from build123d import *

# Parameters (mm, degrees)
F0_R     = 25.4
F0_R_2   = 12.7
F1_DEPTH = 3.175
F2_R     = 12.7
F3_DEPTH = 12.7
F4_R     = 7.9375
F5_DEPTH = 76.2
F7_DEPTH = 25.4
F9_DEPTH = 50.8


with BuildPart() as f1:
    # F0 (on Front) → F1 (new body)
    with BuildSketch(Plane.XZ):
        Circle(F0_R)
        Circle(F0_R_2, mode=Mode.SUBTRACT)
    extrude(amount=F1_DEPTH)

    # F2 (on Front) → F3 (join)
    with BuildSketch(Plane.XZ):
        Circle(F2_R)
    extrude(amount=F3_DEPTH)

    # F4 (on Front) → F5 (cut)
    with BuildSketch(Plane.XZ):
        Circle(F4_R)
    extrude(amount=F5_DEPTH, mode=Mode.SUBTRACT)

    # F6 (on Front) → F7 (cut)
    with BuildSketch(Plane.XZ):
        with BuildLine():
            Line((-0.1134674759, 18.3305198635), (1.9560859375, 17.1526827645))
            ThreePointArc((1.9560859375, 17.1526827645), (2.1885398686, 17.7213288028), (2.2677825241, 18.3305198635))
            ThreePointArc((2.2677825241, 18.3305198635), (-0.7368962138, 20.6287122338), (-2.1682810318, 17.1271525825))
            Line((-2.1682810318, 17.1271525825), (-0.1134674759, 18.3305198635))
        make_face()
        with BuildLine():
            ThreePointArc((-2.1682810318, 17.1271525825), (-0.0987276184, 15.9493154835), (1.9560859375, 17.1526827645))
            Line((1.9560859375, 17.1526827645), (-0.1134674759, 18.3305198635))
            Line((-0.1134674759, 18.3305198635), (-2.1682810318, 17.1271525825))
        make_face()
        with BuildLine():
            Line((-15.9314296043, 9.0669942151), (-13.8766160484, 10.2703614961))
            ThreePointArc((-13.8766160484, 10.2703614961), (-18.0009830177, 10.2448313141), (-15.9166897468, 6.6857898352))
            Line((-15.9166897468, 6.6857898352), (-15.9314296043, 9.0669942151))
        make_face()
        with BuildLine():
            ThreePointArc((-13.5501796043, 9.0669942151), (-13.6332372339, 9.690422953), (-13.8766160484, 10.2703614961))
            Line((-13.8766160484, 10.2703614961), (-15.9314296043, 9.0669942151))
            Line((-15.9314296043, 9.0669942151), (-15.9166897468, 6.6857898352))
            ThreePointArc((-15.9166897468, 6.6857898352), (-14.2424282946, 7.3884156085), (-13.5501796043, 9.0669942151))
        make_face()
        with BuildLine():
            Line((15.8179621284, 9.2635256484), (15.8327019859, 6.8823212684))
            ThreePointArc((15.8327019859, 6.8823212684), (17.5069634381, 7.5849470418), (18.1992121284, 9.2635256484))
            ThreePointArc((18.1992121284, 9.2635256484), (16.4271531891, 11.5655329928), (13.748408715, 10.4413627473))
            Line((13.748408715, 10.4413627473), (15.8179621284, 9.2635256484))
        make_face()
        with BuildLine():
            ThreePointArc((13.748408715, 10.4413627473), (13.7631485725, 8.0601583673), (15.8327019859, 6.8823212684))
            Line((15.8327019859, 6.8823212684), (15.8179621284, 9.2635256484))
            Line((15.8179621284, 9.2635256484), (13.748408715, 10.4413627473))
        make_face()
        with BuildLine():
            ThreePointArc((18.3126796043, -9.0669942151), (17.6100082109, -7.3779929054), (15.9166897468, -6.6857898352))
            Line((15.9166897468, -6.6857898352), (15.9314296043, -9.0669942151))
            Line((15.9314296043, -9.0669942151), (13.8766160484, -10.2703614961))
            ThreePointArc((13.8766160484, -10.2703614961), (16.5548583422, -11.3651865855), (18.3126796043, -9.0669942151))
        make_face()
        with BuildLine():
            Line((15.9314296043, -9.0669942151), (15.9166897468, -6.6857898352))
            ThreePointArc((15.9166897468, -6.6857898352), (13.8618761909, -7.8891571162), (13.8766160484, -10.2703614961))
            Line((13.8766160484, -10.2703614961), (15.9314296043, -9.0669942151))
        make_face()
        with BuildLine():
            ThreePointArc((2.4947174759, -18.3305198635), (2.4116598463, -17.7070911256), (2.1682810318, -17.1271525825))
            Line((2.1682810318, -17.1271525825), (0.1134674759, -18.3305198635))
            Line((0.1134674759, -18.3305198635), (-1.9560859375, -17.1526827645))
            ThreePointArc((-1.9560859375, -17.1526827645), (-0.4957235848, -20.632527208), (2.4947174759, -18.3305198635))
        make_face()
        with BuildLine():
            Line((0.1134674759, -18.3305198635), (2.1682810318, -17.1271525825))
            ThreePointArc((2.1682810318, -17.1271525825), (0.0987276184, -15.9493154835), (-1.9560859375, -17.1526827645))
            Line((-1.9560859375, -17.1526827645), (0.1134674759, -18.3305198635))
        make_face()
        with BuildLine():
            ThreePointArc((-15.8327019859, -6.8823212684), (-17.8727756843, -10.4668929294), (-13.748408715, -10.4413627473))
            Line((-13.748408715, -10.4413627473), (-15.8179621284, -9.2635256484))
            Line((-15.8179621284, -9.2635256484), (-15.8327019859, -6.8823212684))
        make_face()
        with BuildLine():
            Line((-15.8179621284, -9.2635256484), (-13.748408715, -10.4413627473))
            ThreePointArc((-13.748408715, -10.4413627473), (-13.5159547839, -9.8727167091), (-13.4367121284, -9.2635256484))
            ThreePointArc((-13.4367121284, -9.2635256484), (-14.1393835218, -7.5745243387), (-15.8327019859, -6.8823212684))
            Line((-15.8327019859, -6.8823212684), (-15.8179621284, -9.2635256484))
        make_face()
    extrude(amount=F7_DEPTH, mode=Mode.SUBTRACT)

    # F8 (on Front) → F9 (cut)
    with BuildSketch(Plane.XZ):
        with BuildLine():
            ThreePointArc((-4.4252673903, 6.5894548162), (-1.9046648273, 7.7055926538), (0.8456684244, 7.8923222923))
            Line((0.8456684244, 7.8923222923), (-2.026901991, 8.2001204215))
            Line((-2.026901991, 8.2001204215), (-4.4252673903, 6.5894548162))
        make_face()
        with BuildLine():
            ThreePointArc((-7.62557139, 2.203308246), (-6.4121173773, 4.6785314992), (-4.4252673903, 6.5894548162))
            Line((-4.4252673903, 6.5894548162), (-6.8236328118, 4.9787891959))
            Line((-6.8236328118, 4.9787891959), (-7.62557139, 2.203308246))
        make_face()
        with BuildLine():
            ThreePointArc((0.8456684244, 7.8923222923), (3.4940015971, 7.1271213747), (5.7209066054, 5.5022844222))
            Line((5.7209066054, 5.5022844222), (3.7182387979, 7.5845241677))
            Line((3.7182387979, 7.5845241677), (0.8456684244, 7.8923222923))
        make_face()
        with BuildLine():
            ThreePointArc((5.7209066054, 5.5022844222), (7.2577858275, 3.2137907729), (7.919268966, 0.5376665262))
            Line((7.919268966, 0.5376665262), (7.7235743297, 3.4200447632))
            Line((7.7235743297, 3.4200447632), (5.7209066054, 5.5022844222))
        make_face()
        with BuildLine():
            Line((-0.8999415178, -8.3988339591), (1.9046660077, -7.705592362))
            ThreePointArc((1.9046660077, -7.705592362), (-0.8456678406, -7.8923223549), (-3.4940016205, -7.1271213632))
            Line((-3.4940016205, -7.1271213632), (-0.8999415178, -8.3988339591))
        make_face()
        with BuildLine():
            Line((4.7092712059, -7.0123513401), (6.4121173532, -4.6785315323))
            ThreePointArc((6.4121173532, -4.6785315323), (4.4252678659, -6.5894544968), (1.9046660077, -7.705592362))
            Line((1.9046660077, -7.705592362), (4.7092712059, -7.0123513401))
        make_face()
        with BuildLine():
            Line((-8.4275100038, -0.5721728275), (-7.2577857868, -3.2137908648))
            ThreePointArc((-7.2577857868, -3.2137908648), (-7.9192689629, -0.5376665725), (-7.62557139, 2.203308246))
            Line((-7.62557139, 2.203308246), (-8.4275100038, -0.5721728275))
        make_face()
        with BuildLine():
            Line((-6.0880616036, -5.855408826), (-3.4940016205, -7.1271213632))
            ThreePointArc((-3.4940016205, -7.1271213632), (-5.7209065724, -5.5022844564), (-7.2577857868, -3.2137908648))
            Line((-7.2577857868, -3.2137908648), (-6.0880616036, -5.855408826))
        make_face()
        with BuildLine():
            ThreePointArc((7.919268966, 0.5376665262), (7.9329409322, 0.2689877618), (7.9375, 0))
            ThreePointArc((7.9375, 0), (7.5465252846, -2.4604597903), (6.4121173532, -4.6785315323))
            Line((6.4121173532, -4.6785315323), (8.1149635946, -2.3447115955))
            Line((8.1149635946, -2.3447115955), (7.919268966, 0.5376665262))
        make_face()
    extrude(amount=F9_DEPTH, mode=Mode.SUBTRACT)


solid = f1.part
Build history of the part. All positions in model axes, mm. A direction names the side the tool comes from. Round coordinates to 2 decimals unless told otherwise and drop trailing zeros. Write each loop counter-clockwise with the first axis right and the second up, starting at its lowest first coordinate (ties: lowest second). Pieces come first, ordered by that corner, then holes. Notation, with made-up numbers: M 6,6 L 40,6 A24 cw 40,16 Z; hole C 37.5,-34.75 d7. An arc over 180 degrees is marked long. Answer as a JSON object with one key per item and string values. Group by question number.
(1) Flat gauge pins, fed straight in: pin 1 (5 mm diameter, centred on y = -3.5, z = 3.5, fed in from -X); pin 2 (3 mm diameter, centred on x = -6.5, y = -9.5, fed in from +Z); pin 3 (1.5 mm diameter, centred on x = -9, y = -10.5, fed in from +Z). Where does each tip first touch, or does it go through?
(2) Cut at B-B (x = 17.5). Give the cut face in (y, z) (1 decimal).
(3) Cut at C-C (x = 0). Give the cut face in (y, z) (3 decimals), and give its area (3 significant figures).
(4) Cut at A-A (y = -5.75). Give the cut face in (x, z), and give its area (3 significant figures).
(5) Drill centre lines: L1, parallel to Y at x = -19, z = 16 (3 decimals); L2, parallel to X at y = -2.75, z = -3; L3, parallel to X at y = -4.25, z = -3. Where is each one in solid material? Low to high.
(6) Cut at D-D (x = -10.5). Give the cut face in (y, z) (3 decimals), and give its area (3 significant figures).
(7) Which spindle directions (+Z, -Z, +X, -X, +Y, -Y) get a long thin tool onto all of the face, cutting with end or side? Do faces 1 (the flat face through (5, -3.175, 12)), 2 (the flat face through (-6, 0, 6)). Say none if no direction does.
Responses:
{
 "1": {"pin 1": "stops at x = -25.38", "pin 2": "stops at z = 11.67", "pin 3": "stops at z = 9.66"},
 "2": {"outline": "M -3.2,-18.4 L 0,-18.4 L 0,-10.9 L -3.2,-10.9 Z; M -3.2,-7.3 L 0,-7.3 L 0,7.6 L -3.2,7.6 Z; M -3.2,10.9 L 0,10.9 L 0,18.4 L -3.2,18.4 Z"},
 "3": {"outline": "M -12.7,-12.7 L -3.175,-12.7 L -3.175,-15.952 L 0,-15.952 L 0,-8.176 L -12.7,-8.176 Z; M -12.7,7.983 L 0,7.983 L 0,15.952 L -3.175,15.952 L -3.175,12.7 L -12.7,12.7 Z; M -3.175,-25.4 L 0,-25.4 L 0,-20.709 L -3.175,-20.709 Z; M -3.175,20.709 L 0,20.709 L 0,25.4 L -3.175,25.4 Z", "area": "168 mm2"},
 "4": {"outline": "C 0,0 d25.4; hole M -8.43,-0.57 L -6.09,-5.86 L -0.9,-8.4 L 4.71,-7.01 L 8.11,-2.34 L 7.72,3.42 L 3.72,7.58 L -2.03,8.2 L -6.82,4.98 Z", "area": "300 mm2"},
 "5": {"L1": "y = -3.175 to 0", "L2": "x = -25.22 to -7.35, 7.64 to 25.22", "L3": "x = -12.34 to -7.35, 7.64 to 12.34"},
 "6": {"outline": "M -12.7,-7.144 L -3.175,-7.144 L -3.175,-23.128 L 0,-23.128 L 0,23.128 L -3.175,23.128 L -3.175,7.144 L -12.7,7.144 Z", "area": "283 mm2"},
 "7": {"face 1": "-Y", "face 2": "+Z, -Z, +X, -X, +Y"}
}
